Verification items for this drawing (mm, ordinates from the low corner). Coordinates: 2 decimals unless noted, no trailing zeros. Write each loop counter-clockwise with the first axis right and the second up, starting at its lowest first coordinate (ties: lowest second). Pieces come first, ordered by that corner, then holes. Notation, with made-up numbers: (40, 11) -> (79, 11) arc R12 ccw to (79, 21) -> close; hole circle Ø4 at (49.5, 71.25). An arc over 180 degrees is marked (long way). One line per item, written item: value. Start each with the question number.
1) Scan lines: line 1 along Y through (x, z) = (7, 5.5); line 2 along X through (y, z) = (43, 71.5); line 3 along X through (y, z) = (26, 84.5). Record each from-to range of solid material in increasing order. Write a range as [from, to].
2) Sectioned sample at B-B on y = 55.5. Enter the section's corners in (x, z).
3) Draft check along X on the marked faces 1, 2, 3 and 4. Enter one of: +X half, -X half, draft (parallel to the pull), parting line (faces both ways), or undercut.
4) Gauge pin test, flat end, axial feed: P1, Ø2, axis at y = 15.5, z = 25.5, coming from the -X side. Record the tip position at first contact, or that the pin passes through.
5) Sectioned sample at C-C on z = 75. Enter the section's corners in (x, y), plus the area to 3 significant figures.
6) Sectioned sample at D-D on z = 109.5. Enter the section's corners in (x, y), plus the area to 3 significant figures.
7) Sectioned sample at A-A on x = 7. Enter the section's corners in (y, z).
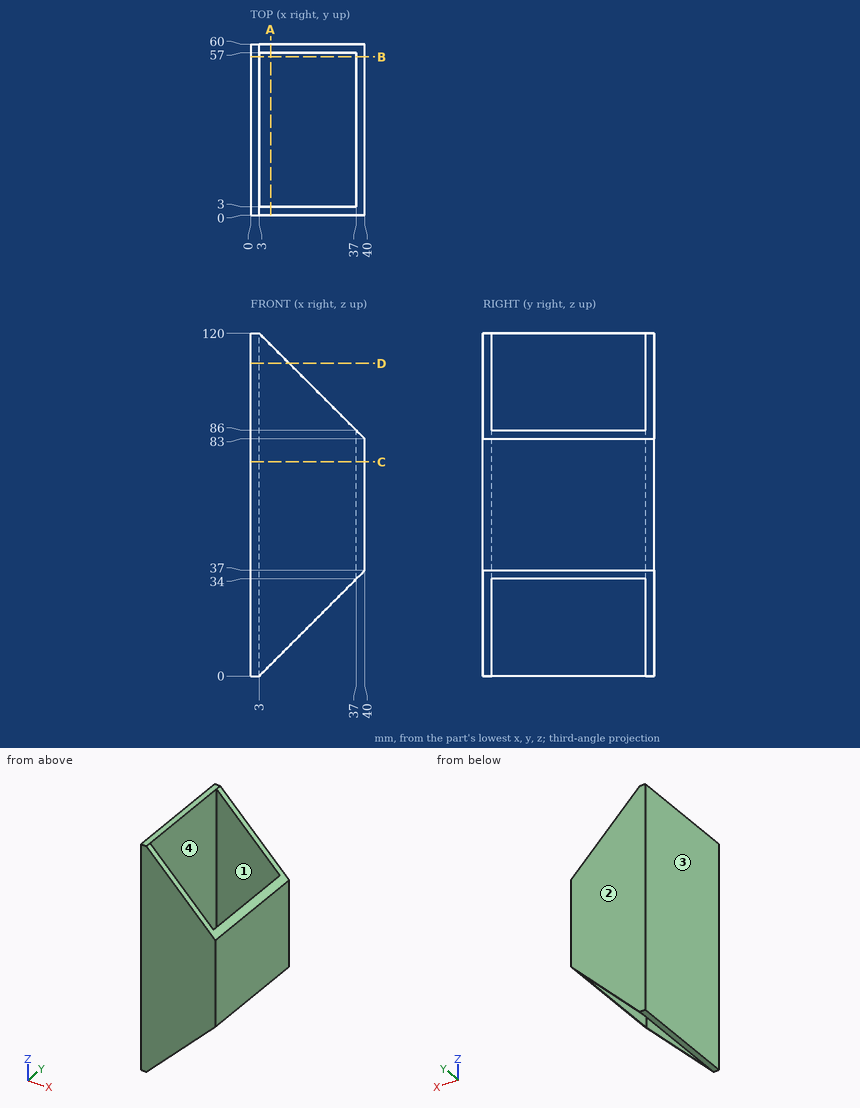
Answers:
1. line 1: y = [0, 3], [57, 60]
1. line 2: x = [0, 3], [37, 40]
1. line 3: x = [0, 3], [37, 38.5]
2. outline: (0, 0) -> (3, 0) -> (3, 120) -> (0, 120) -> close; (37, 34) -> (40, 37) -> (40, 83) -> (37, 86) -> close
3. face 1: undercut
3. face 2: draft
3. face 3: -X half
3. face 4: undercut
4. P1: stops at x = 0
5. outline: (0, 0) -> (40, 0) -> (40, 60) -> (0, 60) -> close; hole (3, 3) -> (37, 3) -> (37, 57) -> (3, 57) -> close
5. area: 564 mm2
6. outline: (0, 0) -> (13.5, 0) -> (13.5, 3) -> (3, 3) -> (3, 57) -> (13.5, 57) -> (13.5, 60) -> (0, 60) -> close
6. area: 243 mm2
7. outline: (0, 4) -> (3, 4) -> (3, 116) -> (0, 116) -> close; (57, 4) -> (60, 4) -> (60, 116) -> (57, 116) -> close
